Autodesk Inventor part; units mm, degrees
ref_plane "Work Plane1" through (30.1625, 0, 0) normal (0, 0, -1) x (1, 0, 0)
ref_plane "YZ Plane" through (0, 0, 0) normal (1, 0, 0) x (0, 1, 0)
ref_plane "XZ Plane" through (0, 0, 0) normal (0, 1, 0) x (-1, 0, 0)
sketch "Rascunho1" plane through (0, 0, 0) normal (0, 0, 1) x (1, 0, 0)
  line L0 (-3.3, 0) -> (20, 0)
  line L1 (20, 0) -> (20, 2.5)
  line L2 (20, 2.5) -> (1.6, 2.5)
  line L3 (1.6, 2.5) -> (1.1091, 2.2547)
  line L4 (1.1091, 2.2547) -> (0, 2.2547)
  line L5 (0, 2.2547) -> (0, 4.25)
  line L6 (-7.96, 0) -> (24.66, 0)
  line L7 (0, -0.85) -> (0, 5.1)
  line L8 (-3.3, 0) -> (-3.3, 3.9613)
  line L9 (0, 4.25) -> (-3.3, 3.9613)
  line L10 (1.6, 2.5) -> (0, 2.5) construction
  dimension "d0" = 20
  dimension "d1" = 18.4
  dimension "d2" = 0.4909
  dimension "d3" = 3.3
  dimension "d4" = 5
  dimension "d5" = 4.5095
  dimension "d9" = 8.5
  dimension "d10" = 5
revolve "Corpo" add sketch "Rascunho1" angle 360 about axis through (-3.3, 0, 0) along (1, 0, 0)
sketch "Rascunho2" plane through (-3.3, 0, 0) normal (-1, 0, 0) x (0, 0, 1)
  circle A0 centre (0, 0) radius 4.25
  line L0 (0, 0) -> (0, 3.9613)
  line L1 (-4.25, 0.755) -> (4.25, 0.755)
  line L2 (4.25, 0.755) -> (4.25, -0.755)
  line L3 (4.25, -0.755) -> (-4.25, -0.755)
  line L4 (-4.25, -0.755) -> (-4.25, 0.755)
  line L5 (-4.25, 0) -> (4.25, 0) construction
  line L6 (0, 0.755) -> (0, -0.755) construction
  point P0 (0, 0)
  dimension "d11" = 1.51
  dimension "d12" = 8.5
fillet "Raio de arredondamento1" radius 0.2 1 edges at (-3.3, -3.9613, 0)
extrude "Fenda" cut sketch "Rascunho2" against normal blind 2 contours A0 L3 L1 | L2 L3 A0 | A0 L1 L2 | A0 L4 L1 | L3 L4 A0
thread "Rosca"
chamfer "Chanfrar1" distance 0.4908 distance2 0.4909 1 edges at (20, -2.5, 0) measured on face at (20, 1.2612, -0.6619)
ref_plane "Work Plane1" through (30.1625, 0, 0) normal (0, 0, -1) x (1, 0, 0)
equation "\"d11\" = SBR"
equation "\"d12\" = KOD"
equation "\"d14\" = RR"
equation "\"d19\" = STI"
equation "\"d15\" = GEL"
equation "\"d17\" = -0.5 * SPD + 0.5 * GD"
equation "\"d0\" = NLG"
equation "\"d1\" = GEL"
equation "\"d3\" = KOH"
equation "\"d4\" = GD"
equation "\"d5\" = BDM"
equation "\"d9\" = KOD"
equation "\"d10\" = KEWI"
equation "\"GD\" = NND"
equation "\"NLG\" = 20"
equation "\"GEL\" = 18.4"
equation "\"KOD\" = 8.5"
equation "\"KOH\" = 3.3"
equation "\"GAL\" = 0.61345 * PTC"
equation "\"SPD\" = NND - 1.2269 * PTC"
equation "\"BDM\" = 4.5095"
equation "\"GUL\" = 0.61345 * PTC"
equation "\"RR\" = 0.2"
equation "\"SBR\" = 1.51"
equation "\"STI\" = 2"
equation "\"KEWI\" = 5deg"
equation "\"PTC\" = 0.8"
equation "\"THREADDIA\" = 5"
equation "\"TOA\" = 30deg"
equation "\"NND\" = 5"
equation "\"GD1\" = THREADDIA - 1.2269 * PTC"
properties part number "BS 4183 - M5 x 20" material "Aço, suave"
Source: CAD feature listing. Evaluate the final solid. Frame: model axes, mm. A direction names the side the tool comes from. Give positions to 0.01 mm unless a question says otherwise; leave off trailing zeros. Loops run counter-clockwise (first coordinate to the right, second up) from the corner with the lowest first, then second, coordinate; pieces in that order, holes last. Notation, with made-up numbers: (47, 17) -> (56, 17) arc R16 ccw to (56, 30) -> close; hole circle Ø3 at (77.5, 63). An arc over 180 degrees is marked (long way). Use a Markdown table: item, result. Add a question column.
1) Reachability of faces 1 (the face through (20, 0, 0)), 2 (the face through (10.43, -0.54, 2.44)), 3 (the face through (0.55, -1.79, 1.37)), 4 (the face through (-3.3, -2, 0)), 5 (the face through (-2, -0.755, 0)) from +Z, -Z, +X, -X, +Y, -Y: full face, straight path, thin tool, end or side. Return the list, or none.
2) Section query A-A, the plane y = 0. Return the cut outline in (x, z).
3) Section query B-B, the plane z = 0. Return the cut outline in (x, y) (3 decimals).
4) First-contact query: pin 1 (1.5 mm diameter, centred on x = 8.5, y = 0.5, fed in from +Z); pin 2 (2.5 mm diameter, centred on y = 2, z = 0.5, fed in from +X); pin 3 (2 mm diameter, centred on x = 12.5, y = -0.5, fed in from -Z); pin 4 (5 mm diameter, centred on x = 8.5, z = 0.5, fed in from +Y). Flat tips, straight axial feed; report the tip coordinate or a pass-through.
5) Line query: line 1 along X through (y, z) = (-0.25, -0.5); line 2 along X through (y, z) = (3.25, 1.25); line 3 along Z through (x, y) = (5, 1). Output: solid intervals per line, ascending. Write a range as [from, to].
6) Section query C-C, the plane x = 12.75. Return the cut outline in (y, z), then the cut area to 3 significant figures.
7) Pull-direction query (Y, two-part tool) for faces 6 (the face through (-1.3, 0, 0)), 7 (the face through (-3.3, 2, 0)), 8 (the face through (-1.88, 1.89, -3.62)); classes: +Y half, -Y half, draft (parallel to the pull), parting line (faces both ways), or undercut.
Numbers:
| question | item | result |
|---|---|---|
| 1 | face 1 | +Z, -Z, +X, +Y, -Y |
| 1 | face 2 | +X |
| 1 | face 3 | none |
| 1 | face 4 | +Z, -Z, -X, +Y, -Y |
| 1 | face 5 | +Z, -Z, -X |
| 2 | outline | (-1.3, -4.14) -> (0, -4.25) -> (0, -2.25) -> (1.11, -2.25) -> (1.6, -2.5) -> (19.51, -2.5) -> (20, -2.01) -> (20, 2.01) -> (19.51, 2.5) -> (1.6, 2.5) -> (1.11, 2.25) -> (0, 2.25) -> (0, 4.25) -> (-1.3, 4.14) -> close |
| 3 | outline | (-3.3, -3.778) arc R0.2 ccw to (-3.117, -3.977) -> (0, -4.25) -> (0, -2.255) -> (1.109, -2.255) -> (1.6, -2.5) -> (19.509, -2.5) -> (20, -2.009) -> (20, 2.009) -> (19.509, 2.5) -> (1.6, 2.5) -> (1.109, 2.255) -> (0, 2.255) -> (0, 4.25) -> (-3.117, 3.977) arc R0.2 ccw to (-3.3, 3.778) -> (-3.3, 0.755) -> (-1.3, 0.755) -> (-1.3, -0.755) -> (-3.3, -0.755) -> close |
| 4 | pin 1 | stops at z = 2.5 |
| 4 | pin 2 | stops at x = 20 |
| 4 | pin 3 | stops at z = -2.5 |
| 4 | pin 4 | stops at y = 2.5 |
| 5 | line 1 | x = [-1.3, 20] |
| 5 | line 2 | x = [-3.3, 0] |
| 5 | line 3 | z = [-2.29, 2.29] |
| 6 | outline | circle Ø5 at (0, 0) |
| 6 | area | 19.6 mm2 |
| 7 | face 6 | undercut |
| 7 | face 7 | draft |
| 7 | face 8 | parting line |
